```python
from build123d import *

# Parameters (mm, degrees)
SKETCH2_W           = 28.2
SKETCH2_H           = 28.2
BOSS_EXTRUDE1_DEPTH = 5
SKETCH3_R           = 1.4
CUT_EXTRUDE1_DEPTH  = 5
SKETCH4_R           = 11.5
CUT_EXTRUDE2_DEPTH  = 5
SKETCH7_W           = 55
SKETCH7_H           = 28.2
BOSS_EXTRUDE2_DEPTH = 3
SKETCH10_R          = 1.6
CUT_EXTRUDE7_DEPTH  = 5


with BuildPart() as part:
    # Sketch2 → Boss-Extrude1 (new body)
    with BuildSketch(Plane.XY):
        with Locations((17.317401284, 44.516795377)):
            Rectangle(SKETCH2_W, SKETCH2_H)
    extrude(amount=BOSS_EXTRUDE1_DEPTH)

    # Sketch3 → Cut-Extrude1 (cut)
    with BuildSketch(Plane.XY.offset(5)):
        with Locations((5.817401284, 56.016795377)):
            Circle(SKETCH3_R)
        with Locations((28.817401284, 56.016795377)):
            Circle(SKETCH3_R)
        with Locations((28.817401284, 33.016795377)):
            Circle(SKETCH3_R)
        with Locations((5.817401284, 33.016795377)):
            Circle(SKETCH3_R)
    extrude(amount=-CUT_EXTRUDE1_DEPTH, mode=Mode.SUBTRACT)

    # Sketch4 → Cut-Extrude2 (cut)
    with BuildSketch(Plane.XY.offset(5)):
        with Locations((17.317401284, 44.516795377)):
            Circle(SKETCH4_R)
    extrude(amount=-CUT_EXTRUDE2_DEPTH, mode=Mode.SUBTRACT)

    # Sketch7 → Boss-Extrude2 (add)
    with BuildSketch(Plane.ZY.offset(-3.217401284)):
        with Locations((-12.5, 44.516795377)):
            Rectangle(SKETCH7_W, SKETCH7_H)
    extrude(amount=BOSS_EXTRUDE2_DEPTH)

    # Sketch10 → Cut-Extrude7 (cut)
    with BuildSketch(Plane(origin=(3.217401284, 0, 0), x_dir=(0, 0, -1), z_dir=(1, 0, 0))):
        with Locations(Location((37, 55.616795377, 0), (0, 0, 90))):
            Circle(SKETCH10_R)
        with Locations(Location((37, 33.416795377, 0), (0, 0, 90))):
            Circle(SKETCH10_R)
        with Locations(Location((-12, 55.616795377, 0), (0, 0, 90))):
            Circle(SKETCH10_R)
        with Locations(Location((-12, 33.416795377, 0), (0, 0, 90))):
            Circle(SKETCH10_R)
    extrude(amount=-CUT_EXTRUDE7_DEPTH, mode=Mode.SUBTRACT)


solid = part.part
```
The model under review builds one solid part; all positions refer to its coordinate system, in mm. A direction names the side the tool comes from. Round coordinates to 2 decimals unless told otherwise and drop trailing zeros. Loops run counter-clockwise (first coordinate to the right, second up) from the corner with the lowest first, then second, coordinate; pieces in that order, holes last.
1) Consider section A-A on z = 12. State the section outline as (x, y) points, then the cut area to 3 significant figures.
Values follow:
outline: (0.22, 30.42) - (3.22, 30.42) - (3.22, 31.82) - (0.22, 31.82) - close; (0.22, 35.02) - (3.22, 35.02) - (3.22, 54.02) - (0.22, 54.02) - close; (0.22, 57.22) - (3.22, 57.22) - (3.22, 58.62) - (0.22, 58.62) - close
area: 65.4 mm2
2) Clearance check with flat-ended pins moving along their axes: P1, Ø3.5, axis at x = 5.82, y = 33.02, coming from the +Z side; P2, Ø3, axis at x = 28.82, y = 33.02, coming from the -Z side; P3, Ø4, axis at y = 33.42, z = 12, coming from the +X side. State where each tip first meets the part, or that it passes through.
Values follow:
P1: stops at z = 5
P2: stops at z = 0
P3: stops at x = 3.22
3) The part is to be moulded in two halves that separate along Y. For faces 4 (the face through (3, 58.617, -7)), 5 (the face through (0.217, 45, -13)), 6 (the face through (27.71, 32.16, 2.54)), say which applies: pulls with the +Y half, pulls with the -Y half, needs draft (parallel to the pull), parting line crosses it, or undercut.
Values follow:
face 4: pulls with the +Y half
face 5: needs draft
face 6: undercut
4) Wall thickness on line 1 along X through (y, z) = (51, -32); line 2 along Z through (x, y) = (24.5, 56); line 3 along X through (y, z) = (35.75, 4): over which ranges is each line inside the solid? List them lowest first.
Values follow:
line 1: x = 0.22 to 3.22
line 2: z = 0 to 5
line 3: x = 0.22 to 9.87, 24.76 to 31.42
5) Tool access review of faces 1 (the face through (3.217, 45, -20)), 2 (the face through (1.7, 34.9, -37.6)), 3 (the face through (17, 57, 5)): name each direction out of +Z, -Z, +X, -X, +Y, -Y from which nothing blocks a thin tool from reaching the whole face with its end or side.
Values follow:
face 1: -Z, +X, +Y, -Y
face 2: +X, -X
face 3: +Z, +X, +Y, -Y
6) Consider section B-B on y = 35.75. State the section outline as (x, z) points, then the cut area to 3 significant figures.
Values follow:
outline: (0.22, -40) - (3.22, -40) - (3.22, 0) - (9.87, 0) - (9.87, 5) - (3.22, 5) - (3.22, 15) - (0.22, 15) - close; (24.76, 0) - (31.42, 0) - (31.42, 5) - (24.76, 5) - close
area: 232 mm2
7) Consider section C-C on x = 17.5. State the section outline as (y, z) points.
Values follow:
outline: (30.42, 0) - (33.02, 0) - (33.02, 5) - (30.42, 5) - close; (56.02, 0) - (58.62, 0) - (58.62, 5) - (56.02, 5) - close
8) Consider section D-D on z = 2.5. State the section outline as (x, y) points, then the cut area to 3 significant figures.
Values follow:
outline: (0.22, 30.42) - (31.42, 30.42) - (31.42, 58.62) - (0.22, 58.62) - close; hole circle Ø2.8 at (5.82, 33.02); hole circle Ø2.8 at (5.82, 56.02); hole circle Ø23 at (17.32, 44.52); hole circle Ø2.8 at (28.82, 33.02); hole circle Ø2.8 at (28.82, 56.02)
area: 440 mm2
